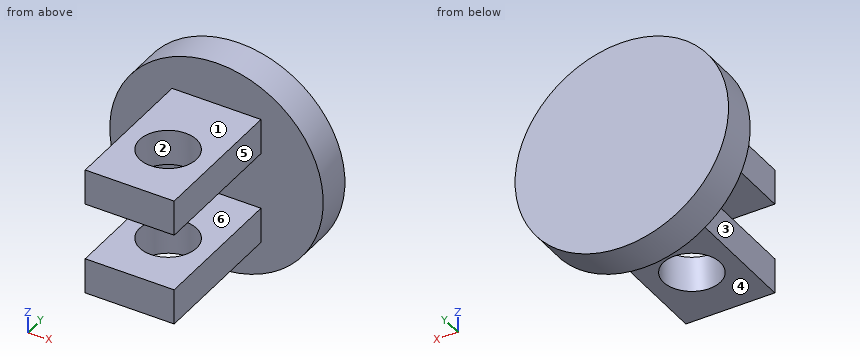
from build123d import *

# Parameters (mm, degrees)
SKETCH_1_R          = 6
SKETCH_1_W          = 5
SKETCH_1_H          = 2
EXTRUDE_1_DEPTH     = 2
SKETCH_1_3_W        = 5
SKETCH_1_3_H        = 2
EXTRUDE_2_DEPTH     = 8
SKETCH_2_R          = 1.6
CUT_EXTRUDE_1_DEPTH = 14.862178761


with BuildPart() as part:
    # Sketch 1 → Extrude 1 (new body)
    # profile 1 of 3: a face of its own
    with BuildSketch(Plane(origin=(0, 0, 0), x_dir=(1, 0, 0), z_dir=(0, 1, 0))):
        with Locations(Location((0, 0, 0), (0, 0, 270))):
            Circle(SKETCH_1_R)
        with Locations((0, -2.6)):
            Rectangle(SKETCH_1_W, SKETCH_1_H, mode=Mode.SUBTRACT)
        with Locations((0, 2.6)):
            Rectangle(SKETCH_1_W, SKETCH_1_H, mode=Mode.SUBTRACT)
    # profile 2 of 3: a face of its own
    with BuildSketch(Plane(origin=(0, 0, 0), x_dir=(1, 0, 0), z_dir=(0, 1, 0))):
        with Locations((0, 2.6)):
            Rectangle(SKETCH_1_W, SKETCH_1_H)
    # profile 3 of 3: a face of its own
    with BuildSketch(Plane(origin=(0, 0, 0), x_dir=(1, 0, 0), z_dir=(0, 1, 0))):
        with Locations((0, -2.6)):
            Rectangle(SKETCH_1_W, SKETCH_1_H)
    extrude(amount=EXTRUDE_1_DEPTH)

    # Sketch 1_3 → Extrude 2 (add)
    with BuildSketch(Plane(origin=(0, 0, 0), x_dir=(1, 0, 0), z_dir=(0, 1, 0))):
        with Locations((0, 2.6)):
            Rectangle(SKETCH_1_3_W, SKETCH_1_3_H)
        with Locations((0, -2.6)):
            Rectangle(SKETCH_1_3_W, SKETCH_1_3_H)
    extrude(amount=-EXTRUDE_2_DEPTH)

    # Sketch 2 → Cut-Extrude 1 (cut, through all)
    with BuildSketch(Plane.XY.offset(3.6)):
        with Locations((0, -4.46004136)):
            Circle(SKETCH_2_R)
    extrude(amount=-CUT_EXTRUDE_1_DEPTH, mode=Mode.SUBTRACT)


solid = part.part
Input: part model. Units: mm. Frame: model coordinates. Face numbers are marked on the shaded views. A direction names the side the tool comes from. Coordinates: 2 decimals unless noted, no trailing zeros. Loops run counter-clockwise (first coordinate to the right, second up) from the corner with the lowest first, then second, coordinate; pieces in that order, holes last.
Q1. Cut plane B-B (y = -1.25). Output: boundary loops of the cut face in (x, z), then the cut area to 3 significant figures.
Q2. Draft query along X for the marked faces 1, 2 and 3. Return one class per face: +X half, -X half, draft (parallel to the pull), parting line (faces both ways), or undercut.
Q3. Material intervals for line 1 (Y direction, x = 0, z = -2.9); line 2 (Z direction, x = -2.25, y = -0.5); line 3 (X direction, y = -7, z = 2.25), sorted ascending.
Q4. Set-up query: the marked faces 4, 5 and 6. Return all of +Z, -Z, +X, -X, +Y, -Y with unobstructed straight access to the full face (end or side cutting, diameter ignored); none if empty.
Q5. Cut plane C-C (y = -3.5). Output: boundary loops of the cut face in (x, z), then the cut area to 3 significant figures.
Q6. Contact query for flat-ended pins moving along their axis: pin 1 (4 mm diameter, centred on x = 0.5, y = -3, fed in from -Z); pin 2 (2 mm diameter, centred on y = -2.5, z = 3, fed in from -X); pin 3 (1.6 mm diameter, centred on y = -4.5, z = -3, fed in from +X). Output: stop coordinate, or through.
Q7. Cut plane D-D (z = 2.5). Output: boundary loops of the cut face in (x, y).
Q8. Cut plane A-A (x = 0). Output: boundary loops of the cut face in (y, z), then the cut area to 3 significant figures.
Working result:
1. outline: (-2.5, -3.6) - (2.5, -3.6) - (2.5, -1.6) - (-2.5, -1.6) - close; (-2.5, 1.6) - (2.5, 1.6) - (2.5, 3.6) - (-2.5, 3.6) - close
1. area: 20.0 mm2
2. face 1: draft
2. face 2: undercut
2. face 3: -X half
3. line 1: y = -8 to -6.06, -2.86 to 2
3. line 2: z = -3.6 to -1.6, 1.6 to 3.6
3. line 3: x = -2.5 to 2.5
4. face 4: -Z, +X, -X, -Y
4. face 5: +Z, -Z, +X, -Y
4. face 6: +X, -X, -Y
5. outline: (-2.5, -3.6) - (-1.28, -3.6) - (-1.28, -1.6) - (-2.5, -1.6) - close; (-2.5, 1.6) - (-1.28, 1.6) - (-1.28, 3.6) - (-2.5, 3.6) - close; (1.28, -3.6) - (2.5, -3.6) - (2.5, -1.6) - (1.28, -1.6) - close; (1.28, 1.6) - (2.5, 1.6) - (2.5, 3.6) - (1.28, 3.6) - close
5. area: 9.76 mm2
6. pin 1: stops at z = -3.6
6. pin 2: stops at x = -2.5
6. pin 3: stops at x = 2.5
7. outline: (-5.45, 0) - (-2.5, 0) - (-2.5, -8) - (2.5, -8) - (2.5, 0) - (5.45, 0) - (5.45, 2) - (-5.45, 2) - close; hole circle Ø3.2 at (0, -4.46)
8. outline: (-8, -3.6) - (-6.06, -3.6) - (-6.06, -1.6) - (-8, -1.6) - close; (-8, 1.6) - (-6.06, 1.6) - (-6.06, 3.6) - (-8, 3.6) - close; (-2.86, -3.6) - (0, -3.6) - (0, -6) - (2, -6) - (2, 6) - (0, 6) - (0, 3.6) - (-2.86, 3.6) - (-2.86, 1.6) - (0, 1.6) - (0, -1.6) - (-2.86, -1.6) - close
8. area: 43.2 mm2
